from build123d import *

# Parameters (mm, degrees)
SKETCH_1_W          = 2.8
SKETCH_1_H          = 2.8
EXTRUDE_1_DEPTH     = 4.5
SKETCH_2_W          = 9
SKETCH_2_H          = 24
EXTRUDE_2_DEPTH     = 2
SKETCH_3_W          = 24
SKETCH_3_H          = 31.3
EXTRUDE_3_DEPTH     = 1
SKETCH_3_3_W        = 20
SKETCH_3_3_H        = 7.433333333
SKETCH_3_3_H_2      = 9.433333334
SKETCH_3_3_H_3      = 9.433333333
CUT_EXTRUDE_1_DEPTH = 35.708644456
SKETCH_3_4_W        = 2
SKETCH_3_4_H        = 7.433333333
SKETCH_3_4_H_2      = 1.5
SKETCH_3_4_H_3      = 9.433333334
SKETCH_3_4_H_4      = 9.433333333
SKETCH_3_4_H_5      = 2
EXTRUDE_4_DEPTH     = 10
SKETCH_5_W          = 19
SKETCH_5_H          = 2
SKETCH_5_W_2        = 14.5
EXTRUDE_5_DEPTH     = 25.5
SKETCH_6_W          = 6.5
SKETCH_6_H          = 12.2
CUT_EXTRUDE_2_DEPTH = 43.563951884


with BuildPart() as part:
    # Sketch 1 → Extrude 1 (new body)
    with BuildSketch(Plane(origin=(0, 0, 0), x_dir=(1, 0, 0), z_dir=(0, 1, 0))):
        Rectangle(SKETCH_1_W, SKETCH_1_H)
    extrude(amount=EXTRUDE_1_DEPTH)

    # Sketch 2 → Extrude 2 (add)
    with BuildSketch(Plane.XZ):
        with Locations((-1.5, 0)):
            Rectangle(SKETCH_2_W, SKETCH_2_H)
    extrude(amount=-EXTRUDE_2_DEPTH)

    # Sketch 3 → Extrude 3 (add)
    with BuildSketch(Plane.ZY.offset(6)):
        with Locations((0, 15.65)):
            Rectangle(SKETCH_3_W, SKETCH_3_H)
    extrude(amount=EXTRUDE_3_DEPTH)

    # Sketch 3_3 → Cut-Extrude 1 (cut, through all)
    with BuildSketch(Plane.ZY.offset(6)):
        with Locations((0, 5.716666667)):
            Rectangle(SKETCH_3_3_W, SKETCH_3_3_H)
        with Locations((0, 15.65)):
            Rectangle(SKETCH_3_3_W, SKETCH_3_3_H_2)
        with Locations((0, 26.583333334)):
            Rectangle(SKETCH_3_3_W, SKETCH_3_3_H_3)
    extrude(amount=CUT_EXTRUDE_1_DEPTH, mode=Mode.SUBTRACT)

    # Sketch 3_4 → Extrude 4 (add)
    with BuildSketch(Plane.ZY.offset(6)):
        with Locations((11, 5.716666667)):
            Rectangle(SKETCH_3_4_W, SKETCH_3_4_H)
        with Locations((11, 10.183333333)):
            Rectangle(SKETCH_3_4_W, SKETCH_3_4_H_2)
        with Locations((11, 15.65)):
            Rectangle(SKETCH_3_4_W, SKETCH_3_4_H_3)
        with Locations((11, 21.116666667)):
            Rectangle(SKETCH_3_4_W, SKETCH_3_4_H_2)
        with Locations((11, 26.583333334)):
            Rectangle(SKETCH_3_4_W, SKETCH_3_4_H_4)
        with Locations((-11, 26.583333334)):
            Rectangle(SKETCH_3_4_W, SKETCH_3_4_H_4)
        with Locations((-11, 21.116666667)):
            Rectangle(SKETCH_3_4_W, SKETCH_3_4_H_2)
        with Locations((-11, 15.65)):
            Rectangle(SKETCH_3_4_W, SKETCH_3_4_H_3)
        with Locations((-11, 10.183333333)):
            Rectangle(SKETCH_3_4_W, SKETCH_3_4_H_2)
        with Locations((-11, 5.716666667)):
            Rectangle(SKETCH_3_4_W, SKETCH_3_4_H)
        with Locations((11, 1)):
            Rectangle(SKETCH_3_4_W, SKETCH_3_4_H_5)
        with Locations((-11, 1)):
            Rectangle(SKETCH_3_4_W, SKETCH_3_4_H_5)
    extrude(amount=EXTRUDE_4_DEPTH)

    # Sketch 5 → Extrude 5 (add)
    with BuildSketch(Plane.XZ):
        with Locations((-6.5, 11)):
            Rectangle(SKETCH_5_W, SKETCH_5_H)
        with Locations((-8.75, -11)):
            Rectangle(SKETCH_5_W_2, SKETCH_5_H)
    extrude(amount=EXTRUDE_5_DEPTH)

    # Sketch 6 → Cut-Extrude 2 (cut, through all)
    with BuildSketch(Plane(origin=(0, 0, -12), x_dir=(-1, 0, 0), z_dir=(0, 0, -1))):
        with Locations((11.25, -17.9)):
            Rectangle(SKETCH_6_W, SKETCH_6_H)
        with Locations((11.25, -4.2)):
            Rectangle(SKETCH_6_W, SKETCH_6_H)
        with Locations((11.25, 9.5)):
            Rectangle(SKETCH_6_W, SKETCH_6_H)
        with Locations((11.25, 23.2)):
            Rectangle(SKETCH_6_W, SKETCH_6_H)
    extrude(amount=-CUT_EXTRUDE_2_DEPTH, mode=Mode.SUBTRACT)


solid = part.part
Here's how the part is built. I have some questions about the finished solid (model axes, mm). A direction names the side the tool comes from. Coordinates: 2 decimals unless noted, no trailing zeros. Order: outer loops, then holes, each group sorted by start corner. A loop starts at its lowest first (then second) coordinate and runs counter-clockwise, first axis right, second up.
Item 1: If we section it at A-A on y = -21: List the corners of the cut face in (x, z) for me, plus the area to 3 significant figures.
Result sheet:
outline: (-16, -12) - (-14.5, -12) - (-14.5, -10) - (-16, -10) - close; (-16, 10) - (-14.5, 10) - (-14.5, 12) - (-16, 12) - close; (-8, -12) - (-1.5, -12) - (-1.5, -10) - (-8, -10) - close; (-8, 10) - (3, 10) - (3, 12) - (-8, 12) - close
area: 41.0 mm2
Item 2: If we section it at C-C on x = -3.75: List the corners of the cut face in (y, z) for me, plus the area to 3 significant figures.
Result sheet:
outline: (-25.5, -12) - (2, -12) - (2, 12) - (-25.5, 12) - (-25.5, 10) - (0, 10) - (0, -10) - (-25.5, -10) - close
area: 150 mm2
Item 3: If we section it at D-D on y = 8: List the corners of the cut face in (x, z) for me, plus the area to 3 significant figures.
Result sheet:
outline: (-16, -12) - (-14.5, -12) - (-14.5, -10) - (-16, -10) - close; (-16, 10) - (-14.5, 10) - (-14.5, 12) - (-16, 12) - close; (-8, -12) - (-6, -12) - (-6, -10) - (-8, -10) - close; (-8, 10) - (-6, 10) - (-6, 12) - (-8, 12) - close
area: 14.0 mm2
Item 4: For faces 1 (the face through (1.4, 3, 0)), 2 (the face through (-16, 3, -11)), 3 (the face through (-1.4, 3, 0)), 4 (the face through (-14.5, -18, -11)), which set-ups out of +Z, -Z, +X, -X, +Y, -Y let a thin tool reach every point of the face, with its end or its side?
Result sheet:
face 1: +Z, -Z, +X, +Y
face 2: +Z, -Z, -X, +Y, -Y
face 3: +Z, -Z, -X, +Y
face 4: +Z, -Z
Item 5: If we mould it in two halves opening along Z, with no side actions, what happens to faces 5 (the face through (0, 3, 1.4)), 6 (the face through (-6.5, 9.433, -0.1)), 7 (the face through (-7, 21, 0)), 8 (the face through (-8, 9, 11))? For each: +Z half, -Z half, draft (parallel to the pull), parting line (faces both ways), or undercut.
Result sheet:
face 5: +Z half
face 6: undercut
face 7: undercut
face 8: draft
Item 6: I need wall thicknesses on line 1 (Z direction, x = -12, y = 2); line 2 (X direction, y = -7, z = -10.5); line 3 (Y direction, x = 0.75, z = -0.25). Which ranges of each line are inside material? Lowest first, please.
Result sheet:
line 1: z = -12 to -10, 10 to 12
line 2: x = -16 to -14.5, -8 to -1.5
line 3: y = 0 to 4.5
Item 7: For P1, Ø2, axis at y = 1, z = 5, coming from the -X side; P2, Ø2, axis at y = -16, z = -11.5, coming from the +X side; P3, Ø2, axis at x = -1.5, z = 4.5, coming from the -Y side; P4, Ø10, axis at x = -9, y = 7.5, coming from the -Z side, each with a flat end and sliding along its axis, tell me the tip position at first contact or that it passes through.
Result sheet:
P1: stops at x = -7
P2: stops at x = -1.5
P3: stops at y = 0
P4: stops at z = -12
Item 8: If we section it at B-B on z = -7.5: List the corners of the cut face in (x, y) for me.
Result sheet:
outline: (-7, 0) - (3, 0) - (3, 2) - (-7, 2) - close; (-7, 9.43) - (-6, 9.43) - (-6, 10.93) - (-7, 10.93) - close; (-7, 20.37) - (-6, 20.37) - (-6, 21.87) - (-7, 21.87) - close
